Part model, mm, in its own coordinate system. Face numbers are marked on the shaded views. A direction names the side the tool comes from. Round coordinates to 2 decimals unless told otherwise and drop trailing zeros. Loops run counter-clockwise (first coordinate to the right, second up) from the corner with the lowest first, then second, coordinate; pieces in that order, holes last.
(1) Mould opens along X. For the marked faces 1, 2, 3 and 4 say: +X half, -X half, draft (parallel to the pull), parting line (faces both ways), or undercut.
(2) Tool access for the marked faces 5, 6 and 7: list every direction of +Z, -Z, +X, -X, +Y, -Y with a clear straight run to the whole face (end or side of a thin tool).
(3) Probe probe 1 along Y at (x, z) = (-6.5, 1.75); probe 2 along X at (y, z) = (1.45, 0); probe 3 along X at (y, z) = (5.5, -3). List the from-to ranges inside material, lowest first.
(4) Cut at C-C on y = 4.5. List the corners of the cut face in (x, z), then the cut area to 3 significant figures.
(5) Cut at A-A on x = 0. List the corners of the cut face in (y, z).
(6) Cut at D-D on x = -7. List the corners of the cut face in (y, z).
(7) Cut at B-B on z = 0. List the corners of the cut face in (x, y).
(8) Flat gauge pin, fed straight in: pin 1 (5.5 mm diameter, centred on x = 0, z = 0, fed in from -Y). Where does the tip first touch, or does it go through?
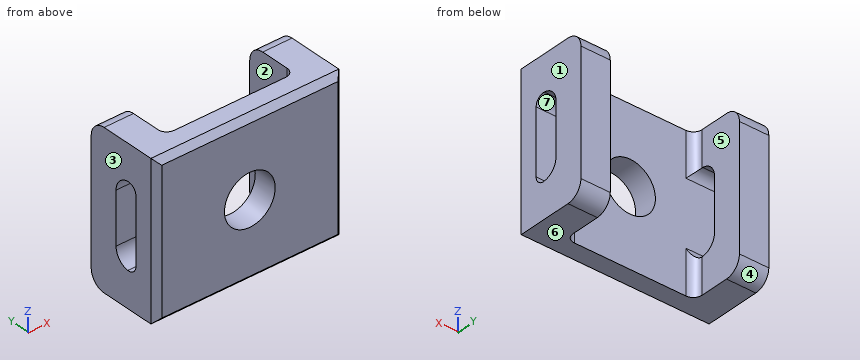
from build123d import *

# Parameters (mm, degrees)
SKETCH1_W               = 16
SKETCH1_H               = 13
SKETCH1_R               = 2.159
BOSS_EXTRUDE1_DEPTH     = 2
BOSS_EXTRUDE2_DEPTH     = 16
CUT_EXTRUDE1_DEPTH      = 17.590660023
CUT_EXTRUDE1_DEPTH_BACK = 17.590660023
SKETCH4_W               = 11
SKETCH4_H               = 5
FILLET1_R               = 0.75
CHAMFER1_SIZE           = 0.5


with BuildPart() as part:
    # Sketch1 → Boss-Extrude1 (new body)
    with BuildSketch(Plane(origin=(0, 0, 0), x_dir=(1, 0, 0), z_dir=(0, 1, 0))):
        Rectangle(SKETCH1_W, SKETCH1_H)
        with Locations(Location((0, 0, 0), (0, 0, 270))):
            Circle(SKETCH1_R, mode=Mode.SUBTRACT)
    extrude(amount=BOSS_EXTRUDE1_DEPTH)

    # Sketch2 → Boss-Extrude2 (add)
    with BuildSketch(Plane(origin=(8, 0, 0), x_dir=(0, 0, -1), z_dir=(1, 0, 0))):
        with BuildLine():
            Line((-6.5, 5.2), (-6.5, 2))
            Line((-6.5, 2), (-3.5, 2))
            Line((-3.5, 2), (-3.5, 2.7))
            ThreePointArc((-3.5, 2.7), (-3.119238816, 3.619238816), (-2.2, 4))
            Line((-2.2, 4), (2.2, 4))
            ThreePointArc((2.2, 4), (3.119238816, 3.619238816), (3.5, 2.7))
            Line((3.5, 2.7), (3.5, 2))
            Line((3.5, 2), (6.5, 2))
            Line((6.5, 2), (6.5, 5.2))
            ThreePointArc((6.5, 5.2), (6.119238816, 6.119238816), (5.2, 6.5))
            Line((5.2, 6.5), (-5.2, 6.5))
            ThreePointArc((-5.2, 6.5), (-6.119238816, 6.119238816), (-6.5, 5.2))
        make_face()
    extrude(amount=-BOSS_EXTRUDE2_DEPTH)

    # Sketch4 → Cut-Extrude1 (cut, two sides: drawn at the far end of the back side and taken through both)
    with BuildSketch(Plane.XY.offset(6.5).offset(-CUT_EXTRUDE1_DEPTH_BACK)):
        with Locations((0, 4.5)):
            Rectangle(SKETCH4_W, SKETCH4_H)
    extrude(amount=CUT_EXTRUDE1_DEPTH + CUT_EXTRUDE1_DEPTH_BACK, mode=Mode.SUBTRACT)

    # Fillet1
    # the kernel refuses this fillet: 0.75 mm, written as the material it adds along each edge
    with BuildSketch(Plane(origin=(-5.5, 2, 3.5), x_dir=(1, 0, 0), z_dir=(0, 0, 1)), Plane(origin=(-5.5, 2, -6.5), x_dir=(1, 0, 0), z_dir=(0, 0, 1))) as fillet1_piece_1:
        with BuildLine():
            CenterArc((FILLET1_R, FILLET1_R), FILLET1_R, 180, 90)
            Line((0, FILLET1_R), (-FILLET1_R * 0.02, FILLET1_R))
            Line((-FILLET1_R * 0.02, FILLET1_R), (-FILLET1_R * 0.02, -FILLET1_R * 0.02))
            Line((-FILLET1_R * 0.02, -FILLET1_R * 0.02), (FILLET1_R, -FILLET1_R * 0.02))
            Line((FILLET1_R, -FILLET1_R * 0.02), (FILLET1_R, 0))
        make_face()
    extrude(amount=3)
    with BuildSketch(Plane(origin=(-5.5, 2, 3.5), x_dir=(0, 0, -1), z_dir=(-1, 0, 0)), Plane(origin=(8, 2, 3.5), x_dir=(0, 0, -1), z_dir=(-1, 0, 0))) as fillet1_piece_2:
        with BuildLine():
            CenterArc((0.752277442, -0.75), FILLET1_R, 90, 95.21590857)
            Line((0.005383046, -0.818181818), (-0.069306394, -0.825))
            ThreePointArc((-0.069306394, -0.825), (-0.075, -0.7), (-0.075, 0))
            Line((-0.075, 0), (0, 0.075))
            Line((0, 0.075), (0.752277442, 0.075))
            Line((0.752277442, 0.075), (0.752277442, 0))
        make_face()
    extrude(amount=2.5)
    with BuildSketch(Plane(origin=(5.5, 2, 6.5), x_dir=(0, 1, 0), z_dir=(0, 0, -1)), Plane(origin=(5.5, 2, -3.5), x_dir=(0, 1, 0), z_dir=(0, 0, -1))) as fillet1_piece_3:
        with BuildLine():
            CenterArc((FILLET1_R, -FILLET1_R), FILLET1_R, 90, 90)
            Line((0, -FILLET1_R), (-FILLET1_R * 0.02, -FILLET1_R))
            Line((-FILLET1_R * 0.02, -FILLET1_R), (-FILLET1_R * 0.02, FILLET1_R * 0.02))
            Line((-FILLET1_R * 0.02, FILLET1_R * 0.02), (FILLET1_R, FILLET1_R * 0.02))
            Line((FILLET1_R, FILLET1_R * 0.02), (FILLET1_R, 0))
        make_face()
    extrude(amount=3)
    with BuildSketch(Plane(origin=(8, 2, -3.5), x_dir=(0, 0, 1), z_dir=(-1, 0, 0)), Plane(origin=(-5.5, 2, -3.5), x_dir=(0, 0, 1), z_dir=(-1, 0, 0))) as fillet1_piece_4:
        with BuildLine():
            CenterArc((0.752277442, 0.75), FILLET1_R, 174.78409143, 95.21590857)
            Line((0.005383046, 0.818181818), (-0.069306394, 0.825))
            ThreePointArc((-0.069306394, 0.825), (-0.075, 0.7), (-0.075, 0))
            Line((-0.075, 0), (0, -0.075))
            Line((0, -0.075), (0.752277442, -0.075))
            Line((0.752277442, -0.075), (0.752277442, 0))
        make_face()
    extrude(amount=2.5)
    with BuildSketch(Plane(origin=(-5.5, 2, 1.625), x_dir=(1, 0, 0), z_dir=(0, 0, 1))) as fillet1_piece_5a_section:
        with BuildLine():
            CenterArc((FILLET1_R, FILLET1_R), FILLET1_R, 180, 90)
            Line((0, FILLET1_R), (-FILLET1_R * 0.02, FILLET1_R))
            Line((-FILLET1_R * 0.02, FILLET1_R), (-FILLET1_R * 0.02, -FILLET1_R * 0.02))
            Line((-FILLET1_R * 0.02, -FILLET1_R * 0.02), (FILLET1_R, -FILLET1_R * 0.02))
            Line((FILLET1_R, -FILLET1_R * 0.02), (FILLET1_R, 0))
        make_face()
    fillet1_piece_5a = extrude(amount=4.875, mode=Mode.PRIVATE)
    fillet1_piece_5a = split(fillet1_piece_5a, bisect_by=Plane(origin=(-5.330203664, 2.169796336, 3.5), z_dir=(0, 0, -1)), keep=Keep.TOP, mode=Mode.PRIVATE)
    with BuildSketch(Plane(origin=(-3.454501184, 2, 3.5), x_dir=(0, 0, -1), z_dir=(-1, 0, 0))) as fillet1_piece_5b_section:
        with BuildLine():
            CenterArc((0.752277442, -0.75), FILLET1_R, 90, 95.21590857)
            Line((0.005383046, -0.818181818), (-0.069306394, -0.825))
            ThreePointArc((-0.069306394, -0.825), (-0.075, -0.7), (-0.075, 0))
            Line((-0.075, 0), (0, 0.075))
            Line((0, 0.075), (0.752277442, 0.075))
            Line((0.752277442, 0.075), (0.752277442, 0))
        make_face()
    fillet1_piece_5b = extrude(amount=4.545498816, mode=Mode.PRIVATE)
    fillet1_piece_5b = split(fillet1_piece_5b, bisect_by=Plane(origin=(-5.5, 2.182819777, 3.341220423), z_dir=(1, 0, 0)), keep=Keep.TOP, mode=Mode.PRIVATE)
    fillet1_piece_5 = fillet1_piece_5a & fillet1_piece_5b
    add(fillet1_piece_5)
    with BuildSketch(Plane(origin=(5.5, 2, 6.5), x_dir=(0, 1, 0), z_dir=(0, 0, -1))) as fillet1_piece_6a_section:
        with BuildLine():
            CenterArc((FILLET1_R, -FILLET1_R), FILLET1_R, 90, 90)
            Line((0, -FILLET1_R), (-FILLET1_R * 0.02, -FILLET1_R))
            Line((-FILLET1_R * 0.02, -FILLET1_R), (-FILLET1_R * 0.02, FILLET1_R * 0.02))
            Line((-FILLET1_R * 0.02, FILLET1_R * 0.02), (FILLET1_R, FILLET1_R * 0.02))
            Line((FILLET1_R, FILLET1_R * 0.02), (FILLET1_R, 0))
        make_face()
    fillet1_piece_6a = extrude(amount=4.875, mode=Mode.PRIVATE)
    fillet1_piece_6a = split(fillet1_piece_6a, bisect_by=Plane(origin=(5.330203664, 2.169796336, 3.5), z_dir=(0, 0, -1)), keep=Keep.TOP, mode=Mode.PRIVATE)
    with BuildSketch(Plane(origin=(8, 2, 3.5), x_dir=(0, 0, -1), z_dir=(-1, 0, 0))) as fillet1_piece_6b_section:
        with BuildLine():
            CenterArc((0.752277442, -0.75), FILLET1_R, 90, 95.21590857)
            Line((0.005383046, -0.818181818), (-0.069306394, -0.825))
            ThreePointArc((-0.069306394, -0.825), (-0.075, -0.7), (-0.075, 0))
            Line((-0.075, 0), (0, 0.075))
            Line((0, 0.075), (0.752277442, 0.075))
            Line((0.752277442, 0.075), (0.752277442, 0))
        make_face()
    fillet1_piece_6b = extrude(amount=4.545498816, mode=Mode.PRIVATE)
    fillet1_piece_6b = split(fillet1_piece_6b, bisect_by=Plane(origin=(5.5, 2.182819777, 3.341220423), z_dir=(-1, 0, 0)), keep=Keep.TOP, mode=Mode.PRIVATE)
    fillet1_piece_6 = fillet1_piece_6a & fillet1_piece_6b
    add(fillet1_piece_6)
    with BuildSketch(Plane(origin=(5.5, 2, -1.625), x_dir=(0, 1, 0), z_dir=(0, 0, -1))) as fillet1_piece_7a_section:
        with BuildLine():
            CenterArc((FILLET1_R, -FILLET1_R), FILLET1_R, 90, 90)
            Line((0, -FILLET1_R), (-FILLET1_R * 0.02, -FILLET1_R))
            Line((-FILLET1_R * 0.02, -FILLET1_R), (-FILLET1_R * 0.02, FILLET1_R * 0.02))
            Line((-FILLET1_R * 0.02, FILLET1_R * 0.02), (FILLET1_R, FILLET1_R * 0.02))
            Line((FILLET1_R, FILLET1_R * 0.02), (FILLET1_R, 0))
        make_face()
    fillet1_piece_7a = extrude(amount=4.875, mode=Mode.PRIVATE)
    fillet1_piece_7a = split(fillet1_piece_7a, bisect_by=Plane(origin=(5.330203664, 2.169796336, -3.5), z_dir=(0, 0, 1)), keep=Keep.TOP, mode=Mode.PRIVATE)
    with BuildSketch(Plane(origin=(8, 2, -3.5), x_dir=(0, 0, 1), z_dir=(-1, 0, 0))) as fillet1_piece_7b_section:
        with BuildLine():
            CenterArc((0.752277442, 0.75), FILLET1_R, 174.78409143, 95.21590857)
            Line((0.005383046, 0.818181818), (-0.069306394, 0.825))
            ThreePointArc((-0.069306394, 0.825), (-0.075, 0.7), (-0.075, 0))
            Line((-0.075, 0), (0, -0.075))
            Line((0, -0.075), (0.752277442, -0.075))
            Line((0.752277442, -0.075), (0.752277442, 0))
        make_face()
    fillet1_piece_7b = extrude(amount=4.545498816, mode=Mode.PRIVATE)
    fillet1_piece_7b = split(fillet1_piece_7b, bisect_by=Plane(origin=(5.5, 2.182819777, -3.341220423), z_dir=(-1, 0, 0)), keep=Keep.TOP, mode=Mode.PRIVATE)
    fillet1_piece_7 = fillet1_piece_7a & fillet1_piece_7b
    add(fillet1_piece_7)
    with BuildSketch(Plane(origin=(-3.454501184, 2, -3.5), x_dir=(0, 0, 1), z_dir=(-1, 0, 0))) as fillet1_piece_8a_section:
        with BuildLine():
            CenterArc((0.752277442, 0.75), FILLET1_R, 174.78409143, 95.21590857)
            Line((0.005383046, 0.818181818), (-0.069306394, 0.825))
            ThreePointArc((-0.069306394, 0.825), (-0.075, 0.7), (-0.075, 0))
            Line((-0.075, 0), (0, -0.075))
            Line((0, -0.075), (0.752277442, -0.075))
            Line((0.752277442, -0.075), (0.752277442, 0))
        make_face()
    fillet1_piece_8a = extrude(amount=4.545498816, mode=Mode.PRIVATE)
    fillet1_piece_8a = split(fillet1_piece_8a, bisect_by=Plane(origin=(-5.5, 2.182819777, -3.341220423), z_dir=(1, 0, 0)), keep=Keep.TOP, mode=Mode.PRIVATE)
    with BuildSketch(Plane(origin=(-5.5, 2, -6.5), x_dir=(1, 0, 0), z_dir=(0, 0, 1))) as fillet1_piece_8b_section:
        with BuildLine():
            CenterArc((FILLET1_R, FILLET1_R), FILLET1_R, 180, 90)
            Line((0, FILLET1_R), (-FILLET1_R * 0.02, FILLET1_R))
            Line((-FILLET1_R * 0.02, FILLET1_R), (-FILLET1_R * 0.02, -FILLET1_R * 0.02))
            Line((-FILLET1_R * 0.02, -FILLET1_R * 0.02), (FILLET1_R, -FILLET1_R * 0.02))
            Line((FILLET1_R, -FILLET1_R * 0.02), (FILLET1_R, 0))
        make_face()
    fillet1_piece_8b = extrude(amount=4.875, mode=Mode.PRIVATE)
    fillet1_piece_8b = split(fillet1_piece_8b, bisect_by=Plane(origin=(-5.330203664, 2.169796336, -3.5), z_dir=(0, 0, 1)), keep=Keep.TOP, mode=Mode.PRIVATE)
    fillet1_piece_8 = fillet1_piece_8a & fillet1_piece_8b
    add(fillet1_piece_8)

    # Chamfer1
    chamfer1_edges = [part.edges().sort_by_distance(p)[0] for p in [
        (0, 0, 6.5),
        (-8, 0, 0),
        (0, 0, -6.5),
        (8, 0, 0),
    ]]
    chamfer(chamfer1_edges, length=CHAMFER1_SIZE)


solid = part.part
Final values:
1. face 1: +X half
1. face 2: undercut
1. face 3: -X half
1. face 4: draft
2. face 5: +Z, -Z, +Y
2. face 6: -Z, +X, -X, +Y, -Y
2. face 7: +X, -X
3. probe 1: y = 0 to 2, 4 to 6.5
3. probe 2: x = -8 to -2.16, 2.16 to 8
3. probe 3: x = -8 to -5.5, 5.5 to 8
4. outline: (-8, -6.5) - (-5.5, -6.5) - (-5.5, 6.5) - (-8, 6.5) - close; (5.5, -6.5) - (8, -6.5) - (8, 6.5) - (5.5, 6.5) - close
4. area: 65.0 mm2
5. outline: (0, -6) - (0.5, -6.5) - (2, -6.5) - (2, -2.16) - (0, -2.16) - close; (0, 2.16) - (2, 2.16) - (2, 6.5) - (0.5, 6.5) - (0, 6) - close
6. outline: (0, -6) - (0.5, -6.5) - (5.2, -6.5) arc R1.3 ccw to (6.5, -5.2) - (6.5, 5.2) arc R1.3 ccw to (5.2, 6.5) - (0.5, 6.5) - (0, 6) - close; hole (2, -2.75) arc R0.75 ccw to (2.82, -3.49) arc R1.3 ccw to (4, -2.2) - (4, 2.2) arc R1.3 ccw to (2.82, 3.49) arc R0.75 ccw to (2, 2.75) - close
7. outline: (-8, 0.5) - (-7.5, 0) - (-2.16, 0) - (-2.16, 2) - (-8, 2) - close; (-8, 4) - (-5.5, 4) - (-5.5, 6.5) - (-8, 6.5) - close; (2.16, 0) - (7.5, 0) - (8, 0.5) - (8, 2) - (2.16, 2) - close; (5.5, 4) - (8, 4) - (8, 6.5) - (5.5, 6.5) - close
8. pin 1: stops at y = 0
